For this review, take the finished solid that the model builds, in its own axes (mm). Coordinates: 2 decimals unless noted, no trailing zeros. Loops run counter-clockwise (first coordinate to the right, second up) from the corner with the lowest first, then second, coordinate; pieces in that order, holes last. Notation, with made-up numbers: (30.25, 73) -> (88.25, 73) arc R25 cw to (88.25, 97) -> close; hole circle Ø8 at (5, 55.25). An arc over 180 degrees is marked (long way). Use a Markdown table: item, result.
from build123d import *

# Parameters (mm, degrees)
F1_DEPTH   = 100
F2_SIZE2   = 1
F2_SIZE    = 5
F2_2_SIZE2 = 1
F2_2_SIZE  = 5
F3_SIZE2   = 5
F3_SIZE    = 1
F3_2_SIZE2 = 5
F3_2_SIZE  = 1
F4_R       = 1
F7_DEPTH   = 25
F8_DEPTH   = 25


with BuildPart() as f1:
    # F0 (on Top) → F1 (new body, symmetric)
    with BuildSketch(Plane.XY):
        with BuildLine():
            Line((-3, 0), (-22, 0))
            Line((-22, 0), (-22, -1.5))
            Line((-22, -1.5), (-10, -1.5))
            Line((-10, -1.5), (-10, -2.9619401321))
            Line((-10, -2.9619401321), (-8.5, -2.9619401321))
            Line((-8.5, -2.9619401321), (-8.5, -1.5))
            Line((-8.5, -1.5), (-2.5606601718, -1.5))
            Line((-2.5606601718, -1.5), (-7.8245233162, -6.7638631444))
            Line((-7.8245233162, -6.7638631444), (-10, -6.7638631444))
            Line((-10, -6.7638631444), (-10, -8.5))
            Line((-10, -8.5), (-22, -8.5))
            Line((-22, -8.5), (-22, -10))
            Line((-22, -10), (-10, -10))
            Line((-10, -10), (-10, -22))
            Line((-10, -22), (-8.5, -22))
            Line((-8.5, -22), (-8.5, -10))
            Line((-8.5, -10), (-6.7638631444, -10))
            Line((-6.7638631444, -10), (-6.7638631444, -7.8245233162))
            Line((-6.7638631444, -7.8245233162), (-1.5, -2.5606601718))
            Line((-1.5, -2.5606601718), (-1.5, -8.5))
            Line((-1.5, -8.5), (-2.9619401321, -8.5))
            Line((-2.9619401321, -8.5), (-2.9619401321, -10))
            Line((-2.9619401321, -10), (-1.5, -10))
            Line((-1.5, -10), (-1.5, -22))
            Line((-1.5, -22), (0, -22))
            Line((0, -22), (0, -3))
            ThreePointArc((0, -3), (-0.8786796564, -0.8786796564), (-3, 0))
        make_face()
    extrude(amount=F1_DEPTH, both=True)

    # F2
    f2_edges = [f1.edges().sort_by_distance(p)[0] for p in [
        (-22, -10, 0),
    ]]
    f2_side = f1.faces().sort_by_distance((-16, -10, 0))[0]
    chamfer(f2_edges, length=F2_SIZE, length2=F2_SIZE2, reference=f2_side)

    # F2#2
    f2_2_edges = [f1.edges().sort_by_distance(p)[0] for p in [
        (0, -22, 0),
    ]]
    f2_2_side = f1.faces().sort_by_distance((0, -12.5, 0))[0]
    chamfer(f2_2_edges, length=F2_2_SIZE, length2=F2_2_SIZE2, reference=f2_2_side)

    # F3
    f3_edges = [f1.edges().sort_by_distance(p)[0] for p in [
        (-22, 0, 0),
    ]]
    f3_side = f1.faces().sort_by_distance((-22, -0.75, 0))[0]
    chamfer(f3_edges, length=F3_SIZE, length2=F3_SIZE2, reference=f3_side)

    # F3#2
    f3_2_edges = [f1.edges().sort_by_distance(p)[0] for p in [
        (-10, -22, 0),
    ]]
    f3_2_side = f1.faces().sort_by_distance((-9.25, -22, 0))[0]
    chamfer(f3_2_edges, length=F3_2_SIZE, length2=F3_2_SIZE2, reference=f3_2_side)

    # F4
    f4_edges = [f1.edges().sort_by_distance(p)[0] for p in [
        (-2.56066, -1.5, 0),
        (-1.5, -2.56066, 0),
        (-6.763863, -7.824523, 0),
        (-7.824523, -6.763863, 0),
        (-1.5, -8.5, 0),
        (-8.5, -1.5, 0),
    ]]
    fillet(f4_edges, radius=F4_R)

    # F5 (on Front) → F7 (cut)
    with BuildSketch(Plane.XZ):
        Polygon((0, 100), (-22, 100), (-22, 78), align=None)
        Polygon((-22, -78), (-22, -100), (0, -100), align=None)
    extrude(amount=F7_DEPTH, mode=Mode.SUBTRACT)

    # F6 (on Right) → F8 (cut)
    with BuildSketch(Plane.YZ):
        Polygon((-22, 78), (0, 100), (-22, 100), align=None)
        Polygon((-22, -100), (0, -100), (-22, -78), align=None)
    extrude(amount=-F8_DEPTH, mode=Mode.SUBTRACT)


solid = f1.part
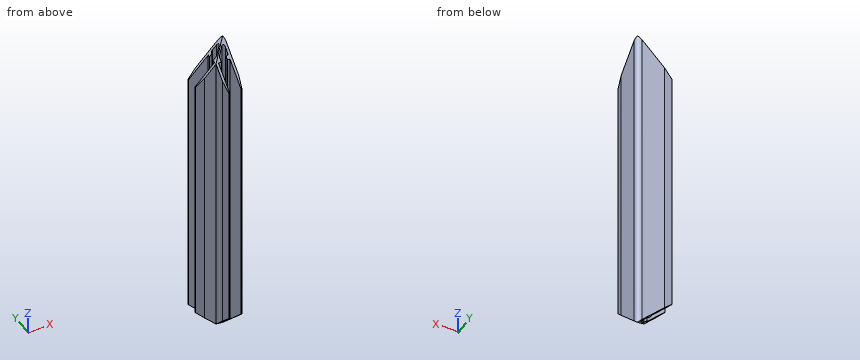
(1) Take a section at A-A on x = -14.75. Write out the cut boundary in (y, z), plus the area to 4 significant figures.
Found:
| item | result |
|---|---|
| outline | (-10, -85.25) -> (-8.5, -85.25) -> (-8.5, 85.25) -> (-10, 85.25) -> close; (-1.5, -85.25) -> (0, -85.25) -> (0, 85.25) -> (-1.5, 85.25) -> close |
| area | 511.5 mm^2 |
(2) For pin 1 Ø2 at (x, z) = (-16.5, 20.5) entering from -Y; pin 2 Ø6 at (x, y) = (-9.5, -18.5) entering from +Z; pin 3 Ø0.5 at (y, z) = (-7.5, 37) entering from -X, all flat-tipped, find the tip position at first contact; note any pin that passes through.
Found:
| item | result |
|---|---|
| pin 1 | stops at y = -10 |
| pin 2 | stops at z = 84.5 |
| pin 3 | stops at x = -10 |
(3) Take a section at B-B on y = -12.5. Write out the cut boundary in (x, z), plus the area to 3 significant figures.
Found:
| item | result |
|---|---|
| outline | (-10, -87.5) -> (-8.5, -87.5) -> (-8.5, 87.5) -> (-10, 87.5) -> close; (-1.5, -87.5) -> (0, -87.5) -> (0, 87.5) -> (-1.5, 87.5) -> close |
| area | 525 mm^2 |
(4) For line 1 along X through (y, z) = (-12.75, -74); line 2 along Y through (x, z) = (-2.75, 2), list the stretches that pass through material, from the lowest coordinate up.
Found:
| item | result |
|---|---|
| line 1 | x = -10 to -8.5, -1.5 to 0 |
| line 2 | y = -10 to -8.5, -4.01 to -0.01 |
